Verification items for the finished model (mm, model axes). Face numbers are marked on the shaded views. A direction names the side the tool comes from. Give positions to 0.01 mm unless a question says otherwise; leave off trailing zeros. Write each loop counter-clockwise with the first axis right and the second up, starting at its lowest first coordinate (ties: lowest second). Pieces come first, ordered by that corner, then holes. Notation, with made-up numbers: M 15.25,-1.5 L 31.25,-1.5 A24 ccw 31.25,14.5 Z; hole C -35.5,-29.5 d5. An arc over 180 degrees is marked long. Write item = value, one per line.
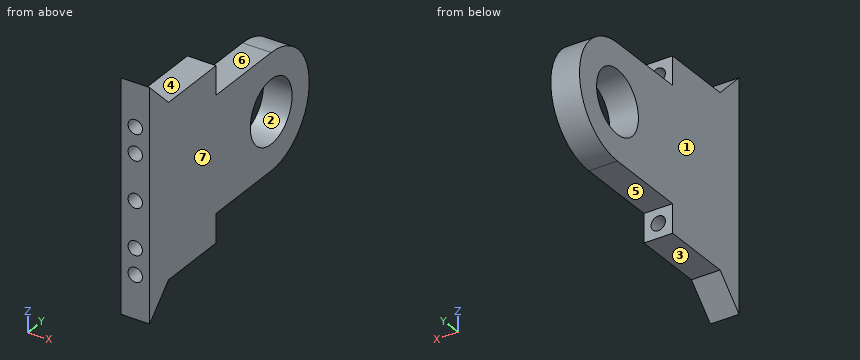
from build123d import *

# Parameters (mm, degrees)
BOSS_EXTRUDE1_DEPTH            = 5
F_11_0_11_DIAMETER_HOLE1_D     = 11
F_11_0_11_DIAMETER_HOLE1_DEPTH = 25
F_11_0_11_DIAMETER_HOLE1_TIP   = 3.304733405
M3_TAPPED_HOLE3_D              = 2.5
M3_TAPPED_HOLE3_DEPTH          = 8
M3_TAPPED_HOLE3_TIP            = 0.751075774


with BuildPart() as part:
    # Sketch1 → Boss-Extrude1 (new body)
    with BuildSketch(Plane(origin=(0, 0, 0), x_dir=(0, 0, -1), z_dir=(1, 0, 0))):
        with BuildLine():
            Line((10, 0), (-10, 0))
            Line((-10, 0), (-20, 0))
            Line((-20, 0), (-15, 5))
            Line((-15, 5), (-15, 10))
            Line((-15, 10), (-15, 17.5))
            Line((-15, 17.5), (-10, 17.5))
            Line((-10, 17.5), (-10, 32))
            ThreePointArc((-10, 32), (0, 42), (10, 32))
            Line((10, 32), (10, 17.5))
            Line((10, 17.5), (15, 17.5))
            Line((15, 17.5), (15, 10))
            Line((15, 10), (15, 5))
            Line((15, 5), (20, 0))
            Line((20, 0), (10, 0))
        make_face()
    extrude(amount=BOSS_EXTRUDE1_DEPTH)

    # Ø11.0 (11) Diameter Hole1
    with Locations(Plane(origin=(0, 32, 0), x_dir=(0, 0, -1), z_dir=(-1, 0, 0))):
        with Locations((0, 0)):
            Hole(F_11_0_11_DIAMETER_HOLE1_D / 2, depth=F_11_0_11_DIAMETER_HOLE1_DEPTH)
            with Locations((0, 0, -(F_11_0_11_DIAMETER_HOLE1_DEPTH + F_11_0_11_DIAMETER_HOLE1_TIP / 2))):  # 118° drill point
                Cone(0, F_11_0_11_DIAMETER_HOLE1_D / 2, F_11_0_11_DIAMETER_HOLE1_TIP, mode=Mode.SUBTRACT)

    # Sketch9 → M3 Tapped Hole2 (revolve, cut)
    with BuildSketch(Plane(origin=(2.5, 17.5, -12.5), x_dir=(0, 0, 1), z_dir=(1, 0, 0))):
        Polygon((0, 0), (0, 18.751075774), (1.25, 18), (1.25, 0), align=None)
    m3_tapped_hole2 = revolve(axis=Axis((2.5, 23.85, -12.5), (0, -1, 0)), mode=Mode.SUBTRACT)

    # Mirror1: M3 Tapped Hole2 across plane
    add(m3_tapped_hole2.mirror(Plane.XY), mode=Mode.SUBTRACT)

    # M3 Tapped Hole3
    with Locations(Plane(origin=(2.5, 0, 8), x_dir=(0, 0, -1), z_dir=(0, -1, 0))):
        with Locations((0, 0), (8, 0), (16, 0)):
            Hole(M3_TAPPED_HOLE3_D / 2, depth=M3_TAPPED_HOLE3_DEPTH)
            with Locations((0, 0, -(M3_TAPPED_HOLE3_DEPTH + M3_TAPPED_HOLE3_TIP / 2))):  # 118° drill point
                Cone(0, M3_TAPPED_HOLE3_D / 2, M3_TAPPED_HOLE3_TIP, mode=Mode.SUBTRACT)


solid = part.part
1) Depth check by flat-ended pin: P1, Ø2, axis at x = 2.5, z = -8, coming from the +Y side; P2, Ø2, axis at x = 2.5, z = -12.5, coming from the -Y side; P3, Ø1.5, axis at x = 1.5, y = 9.5, coming from the +Z side; P4, Ø2.5, axis at x = 3, y = 14.5, coming from the -Z side. Enter the tip coordinate at first touch or a pass-through.
From the geometry:
P1 = 39.14
P2 = through
P3 = 15
P4 = -15
2) Cross-section at B-B on y = 12. Record the boundary of the cut face in (x, z), plus the area to 3 significant figures.
From the geometry:
outline = M 0,-15 L 5,-15 L 5,15 L 0,15 Z; hole C 2.5,-12.5 d2.5; hole C 2.5,12.5 d2.5
area = 140 mm^2
3) Cross-section at D-D on y = 39.5. Record the boundary of the cut face in (x, z).
From the geometry:
outline = M 0,-6.61 L 5,-6.61 L 5,6.61 L 0,6.61 Z
4) Cross-section at C-C on y = 18.5. Record the boundary of the cut face in (x, z).
From the geometry:
outline = M 0,-10 L 5,-10 L 5,10 L 0,10 Z
5) Tool access check on the marked faces 5, 6 and 7. Record the directions out of +Z, -Z, +X, -X, +Y, -Y that give a thin tool (end or side, any length) a straight path to the whole face; none if there is none.
From the geometry:
face_5 = -Z, +X, -X, +Y
face_6 = +Z, +X, -X, +Y
face_7 = +Z, -Z, +X, +Y, -Y
6) Draft check along Z on the marked faces 1, 2, 3 and 4. Enter one of: +Z half, -Z half, draft (parallel to the pull), parting line (faces both ways), or undercut.
From the geometry:
face_1 = draft
face_2 = undercut
face_3 = -Z half
face_4 = +Z half
7) Material ranges on probe 1 along X at (y, z) = (7.75, -12.5); probe 2 along Y at (x, z) = (1.1, 0); probe 3 along Z at (x, y) = (3.45, 32), recorded low to high. Write a range as from..to.
From the geometry:
probe_1 = 0..1.25, 3.75..5
probe_2 = 0..26.5, 37.5..42
probe_3 = -10..-5.5, 5.5..10
8) Cross-section at A-A on z = -12.5. Record the boundary of the cut face in (x, y), plus the area to 4 significant figures.
From the geometry:
outline = M 0,0 L 1.25,0 L 1.25,17.5 L 0,17.5 Z; M 3.75,0 L 5,0 L 5,17.5 L 3.75,17.5 Z
area = 43.75 mm^2
